Work out the finished part from the listing and answer in its coordinate system (mm). Face numbers are marked on the shaded views. Coordinates: 2 decimals unless noted, no trailing zeros. Order: outer loops, then holes, each group sorted by start corner. A loop starts at its lowest first (then second) coordinate and runs counter-clockwise, first axis right, second up.
1. A flat-ended cylindrical pin translates along its axis: pin 1 Ø0.8 at (x, y) = (-50.8, -0.26) entering from -Z. Find the tip coordinate at first contact, or state that the pin passes through.
2. Find the intervals of material crossed by probe 1 along Z at (x, y) = (-53, -4); probe 2 along Y at (x, z) = (-23.5, 12); probe 3 along Z at (x, y) = (-21.5, 5), in increasing order.
3. Determine the mould class of the marked faces 1, 2 and 3 for opening direction Z: +Z half, -Z half, draft (parallel to the pull), parting line (faces both ways), or undercut.
4. The part is cut by section D-D, the plane x = -19. Give the vertices of the cut face in (y, z), then the cut area to 3 significant figures.
5. The part is cut by section B-B, the plane x = -25.4. Give the vertices of the cut face in (y, z).
6. The part is cut by section A-A, the plane z = 13. Give the vertices of the cut face in (x, y).
7. The part is cut by section C-C, the plane y = 4.5. Give the vertices of the cut face in (x, z).
```python
from build123d import *

# Parameters (mm, degrees)
SKETCH1_W           = 38.1
SKETCH1_H           = 38.1
BOSS_EXTRUDE1_DEPTH = 63.5
SKETCH2_R           = 6.3627
CUT_EXTRUDE1_DEPTH  = 57.15
SKETCH6_R           = 2.0193
CUT_EXTRUDE4_DEPTH  = 12.7
SKETCH7_R           = 0.635
CUT_EXTRUDE5_DEPTH  = 22.86


with BuildPart() as part:
    # Sketch1 → Boss-Extrude1 (new body)
    with BuildSketch(Plane(origin=(0, 0, 0), x_dir=(0, 0, -1), z_dir=(1, 0, 0))):
        with Locations((-5.123793103, -0.262758621)):
            Rectangle(SKETCH1_W, SKETCH1_H)
    extrude(amount=-BOSS_EXTRUDE1_DEPTH)

    # Sketch2 → Cut-Extrude1 (cut)
    with BuildSketch(Plane(origin=(0, 0, 0), x_dir=(0, 0, -1), z_dir=(1, 0, 0))):
        with Locations((-11.473793103, -0.262758621)):
            Circle(SKETCH2_R)
    extrude(amount=-CUT_EXTRUDE1_DEPTH, mode=Mode.SUBTRACT)

    # Sketch6 → Cut-Extrude4 (cut)
    with BuildSketch(Plane(origin=(0, 0, -13.926206897), x_dir=(-1, 0, 0), z_dir=(0, 0, -1))):
        with Locations(Location((25.4, -0.262758621, 0), (0, 0, 90))):
            Circle(SKETCH6_R)
    extrude(amount=-CUT_EXTRUDE4_DEPTH, mode=Mode.SUBTRACT)

    # Sketch7 → Cut-Extrude5 (cut)
    with BuildSketch(Plane(origin=(0, 0, -13.926206897), x_dir=(-1, 0, 0), z_dir=(0, 0, -1))):
        with Locations(Location((50.8, -0.262758621, 0), (0, 0, 90))):
            Circle(SKETCH7_R)
    extrude(amount=-CUT_EXTRUDE5_DEPTH, mode=Mode.SUBTRACT)


solid = part.part
```
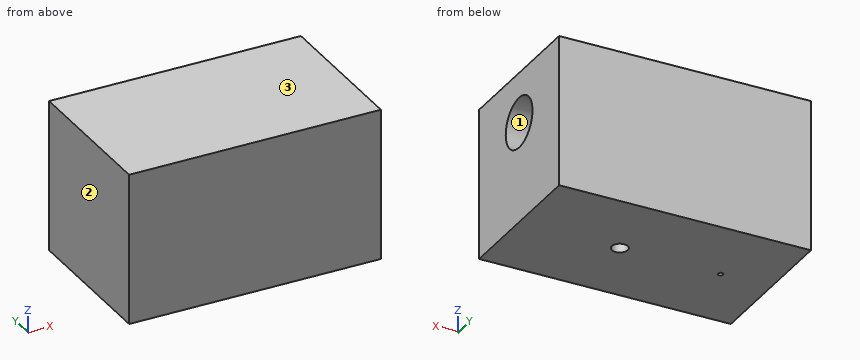
Geometry says:
1. pin 1: stops at z = 17.82
2. probe 1: z = -13.93 to 6.32, 16.62 to 24.17
2. probe 2: y = -19.31 to -6.6, 6.08 to 18.79
2. probe 3: z = -13.93 to 7.9, 15.05 to 24.17
3. face 1: undercut
3. face 2: draft
3. face 3: +Z half
4. outline: (-19.31, -13.93) - (18.79, -13.93) - (18.79, 24.17) - (-19.31, 24.17) - close; hole circle Ø12.73 at (-0.26, 11.47)
4. area: 1,320 mm2
5. outline: (-19.31, -13.93) - (-2.28, -13.93) - (-2.28, -1.23) - (1.76, -1.23) - (1.76, -13.93) - (18.79, -13.93) - (18.79, 24.17) - (-19.31, 24.17) - close; hole circle Ø12.73 at (-0.26, 11.47)
6. outline: (-63.5, -19.31) - (0, -19.31) - (0, -6.44) - (-57.15, -6.44) - (-57.15, 5.91) - (0, 5.91) - (0, 18.79) - (-63.5, 18.79) - close
7. outline: (-63.5, -13.93) - (0, -13.93) - (0, 7.25) - (-57.15, 7.25) - (-57.15, 15.69) - (0, 15.69) - (0, 24.17) - (-63.5, 24.17) - close
